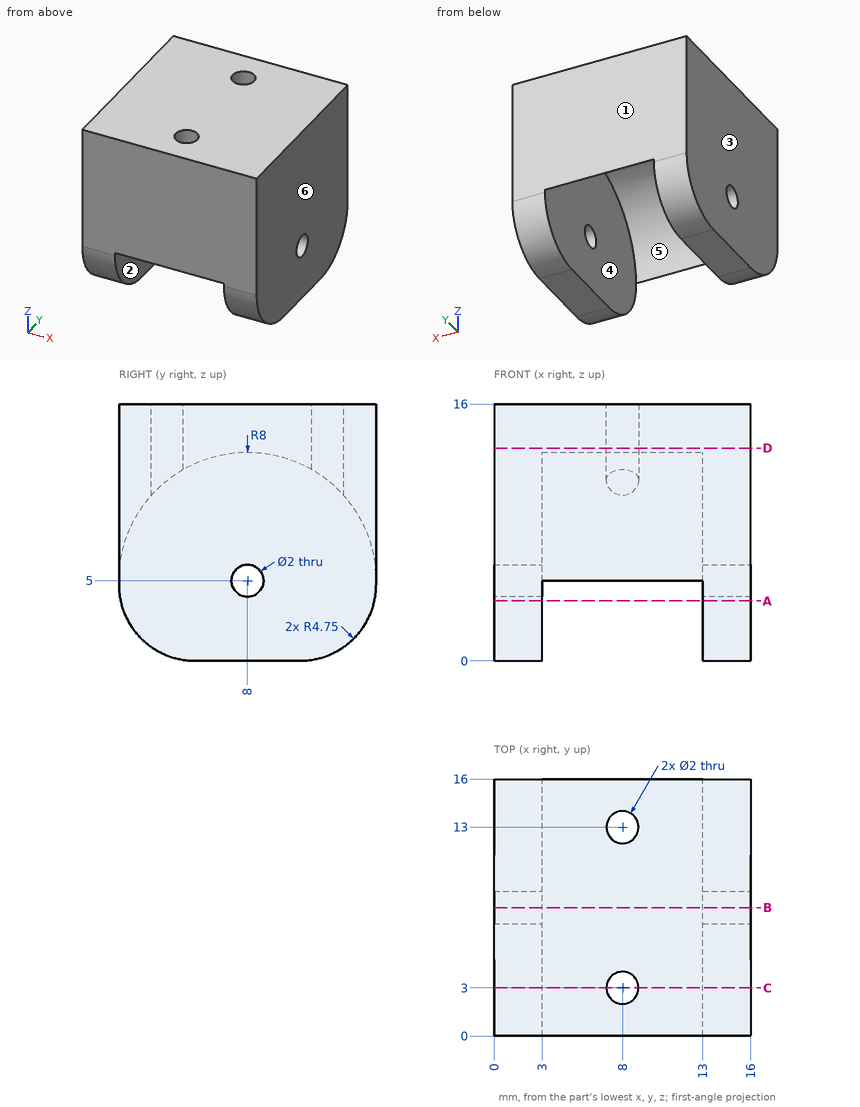
Drawing for the job (mm, zero at the part's lowest x, y, z). A direction names the side the tool comes from. Round coordinates to 2 decimals unless told otherwise and drop trailing zeros. Order: outer loops, then holes, each group sorted by start corner. A loop starts at its lowest first (then second) coordinate and runs counter-clockwise, first axis right, second up.
Item 1: Tool access for the marked faces 1 and 2: list every direction of +Z, -Z, +X, -X, +Y, -Y with a clear straight run to the whole face (end or side of a thin tool).
Item 2: Saw through at C-C on y = 3. Write the cut outline in (x, z) (3 decimals).
Item 3: Saw through at B-B on y = 8. Write the cut outline in (x, z).
Item 4: Saw through at A-A on z = 3.75. Write the cut outline in (x, y).
Item 5: Mould opens along X. For the marked faces 3, 4, 5 and 6 say: pulls with the +X half, pulls with the -X half, needs draft (parallel to the pull), parting line crosses it, or undercut.
Item 6: Saw through at D-D on z = 13.25. Write the cut outline in (x, y).
Item 7: Probe line 1 along Y through (x, z) = (8, 13.3); line 2 along Y through (x, z) = (1.8, 5); line 3 along X through (y, z) = (7.25, 7). List the from-to ranges inside material, lowest first.
Item 8: Pin check, flat tips, straight feed: pin 1 (2 mm diameter, centred on y = 4.5, z = 5, fed in from -X); pin 2 (4 mm diameter, centred on x = 9, y = 7.5, fed in from -Z); pin 3 (2.5 mm diameter, centred on x = 8, y = 3, fed in from -Z). Stop position of each tip, or through.
Reported:
1. face 1: +Z, -Z, +X, -X, +Y
1. face 2: -Z
2. outline: (0, 0.334) - (3, 0.334) - (3, 11.245) - (7, 11.245) - (7, 16) - (0, 16) - close; (9, 11.245) - (13, 11.245) - (13, 0.334) - (16, 0.334) - (16, 16) - (9, 16) - close
3. outline: (0, 0) - (3, 0) - (3, 4) - (0, 4) - close; (0, 6) - (3, 6) - (3, 13) - (13, 13) - (13, 6) - (16, 6) - (16, 16) - (0, 16) - close; (13, 0) - (16, 0) - (16, 4) - (13, 4) - close
4. outline: (0, 0.11) - (3, 0.11) - (3, 15.89) - (0, 15.89) - close; (13, 0.11) - (16, 0.11) - (16, 15.89) - (13, 15.89) - close
5. face 3: pulls with the -X half
5. face 4: undercut
5. face 5: undercut
5. face 6: pulls with the +X half
6. outline: (0, 0) - (16, 0) - (16, 16) - (0, 16) - close; hole circle Ø2 at (8, 3); hole circle Ø2 at (8, 13)
7. line 1: y = 0 to 2, 4 to 12, 14 to 16
7. line 2: y = 0 to 7, 9 to 16
7. line 3: x = 0 to 3, 13 to 16
8. pin 1: stops at x = 0
8. pin 2: stops at z = 12.6
8. pin 3: stops at z = 9.99
